```python
from build123d import *

# Parameters (mm, degrees)
F0_R     = 5
F1_DEPTH = 40
F2_R     = 4.3
F3_DEPTH = 2.25
F4_R     = 5
F5_DEPTH = 6.375
F7_SIZE  = 1
F8_R     = 1.5
F9_DEPTH = 11.53
F10_SIZE = 0.5
F11_SIZE = 5


# Not quite as in the source:
# - a fillet or chamfer that OpenCascade refuses, or shapes differently, is made with other operations: its cross-section is extruded or revolved along the edge and cut away or added


with BuildPart() as f1:
    # F0 (on Front) → F1 (new body)
    with BuildSketch(Plane.XZ):
        Circle(F0_R)
    extrude(amount=F1_DEPTH)

    # F2 (on face) → F3 (join)
    with BuildSketch(Plane(origin=(0, 0, 0), x_dir=(-1, 0, 0), z_dir=(0, 1, 0))):
        Circle(F2_R)
    extrude(amount=F3_DEPTH)

    # F4 (on face) → F5 (join)
    with BuildSketch(Plane(origin=(0, 2.25, 0), x_dir=(-1, 0, 0), z_dir=(0, 1, 0))):
        Circle(F4_R)
    extrude(amount=F5_DEPTH)

    # F6: fillet of radius 1.25 on 3 edges, made by hand

    # F6_s1 → F6_t2 (revolve)
    with BuildSketch(Plane.XY):
        with BuildLine():
            ThreePointArc((-4.3, 1.122497216), (-4.4893398282, 0.4610593883), (-5, 0))
            Line((-5, 0), (-4.3, 0))
            Line((-4.3, 0), (-4.3, 1.122497216))
        make_face()
    revolve(axis=Axis((0, 0, 0), (0, 1, 0)))

    # F6_s3 → F6_t4 (revolve)
    with BuildSketch(Plane.XY):
        with BuildLine():
            ThreePointArc((-5, 2.25), (-4.4893398282, 1.7889406117), (-4.3, 1.127502784))
            Line((-4.3, 1.127502784), (-4.3, 2.25))
            Line((-4.3, 2.25), (-5, 2.25))
        make_face()
    revolve(axis=Axis((0, 2.25, 0), (0, 1, 0)))

    # F7
    f7_edges = [f1.edges().sort_by_distance(p)[0] for p in [
        (5, 8.625, 0),
    ]]
    chamfer(f7_edges, length=F7_SIZE)

    # F8 (on Right) → F9 (join)
    with BuildSketch(Plane.YZ):
        with Locations((-2.875, 0)):
            Circle(F8_R)
    extrude(amount=F9_DEPTH)

    # F10
    f10_edges = [f1.edges().sort_by_distance(p)[0] for p in [
        (11.53, -4.375, 0),
    ]]
    chamfer(f10_edges, length=F10_SIZE)

    # F11
    f11_edges = [f1.edges().sort_by_distance(p)[0] for p in [
        (-5, -40, 0),
    ]]
    chamfer(f11_edges, length=F11_SIZE)


solid = f1.part
```
Here's how the part is built. I have some questions about the finished solid (model axes, mm). A direction names the side the tool comes from. Coordinates: 2 decimals unless noted, no trailing zeros. Loops run counter-clockwise (first coordinate to the right, second up) from the corner with the lowest first, then second, coordinate; pieces in that order, holes last. Notation, with made-up numbers: (35, -15.5) - (40, -15.5) arc R20 cw to (40, -3.5) - close; hole circle Ø1 at (18, 50.5). An arc over 180 degrees is marked (long way). Answer as CSV lines item,"result".
Q1. If I drill on L1, parallel to Z at x = 3, y = -23.5; L2, parallel to Z at x = 1, y = -26; L3, parallel to X at y = -19, z = 2.25, over which ranges is the centre line in solid material (lowest first)? Write a range as [from, to].
Response:
L1,"[-4, 4]"
L2,"[-4.9, 4.9]"
L3,"[-4.47, 4.47]"
Q2. For faces 1 (the face through (0, 8.625, 0)), 2 (the face through (7.856, -1.444, 0.451)), which set-ups out of +Z, -Z, +X, -X, +Y, -Y let a thin tool reach every point of the face, with its end or its side?
Response:
face 1,"+Z, -Z, +X, -X, +Y"
face 2,"+X"
Q3. If we section it at A-A, the plane y = -19: Write out the boundary of the cut face in (x, z).
Response:
outline,"circle Ø10 at (0, 0)"
Q4. If we section it at B-B, the plane x = 10: Write out the boundary of the cut face in (y, z) (3 decimals), and give its area (3 significant figures).
Response:
outline,"circle Ø3 at (-2.875, 0)"
area,"7.07 mm2"
Q5. For pin 1 (1 mm diameter, centred on y = -7, z = 1, fed in from +X); pin 2 (4 mm diameter, centred on x = 5, z = -1.5, fed in from +Y) (3 decimals); pin 3 (1 mm diameter, centred on x = 4, z = -3, fed in from +Y) (3 decimals), each with a flat end and sliding along its axis, tell me the tip position at first contact or that it passes through.
Response:
pin 1,"x = 4.97"
pin 2,"y = 8.625"
pin 3,"y = 8.125"
